Build history of the part. All positions in model axes, mm. Round coordinates to 2 decimals unless told otherwise and drop trailing zeros. Write each loop counter-clockwise with the first axis right and the second up, starting at its lowest first coordinate (ties: lowest second). Pieces come first, ordered by that corner, then holes. Notation, with made-up numbers: (-9, 36) -> (35, 36) arc R34 cw to (35, 73) -> close; hole circle Ø1 at (61.5, -39). An arc over 180 degrees is marked (long way). Answer in a Markdown table with one row per item.
```python
from build123d import *

# Parameters (mm, degrees)
F0_W        = 25.4
F0_H        = 25.4
F1_DEPTH    = 7.62
F2_R        = 5.08
F3_T1_DEPTH = 47.3970452561
F3_T3_DEPTH = 47.3970452561


# Not quite as in the source:
# - a fillet or chamfer that OpenCascade refuses, or shapes differently, is made with other operations: its cross-section is extruded or revolved along the edge and cut away or added


with BuildPart() as f1:
    # F0 (on Front) → F1 (new body)
    with BuildSketch(Plane.XZ):
        Rectangle(F0_W, F0_H)
    extrude(amount=F1_DEPTH)

    # F2
    f2_edges = [f1.edges().sort_by_distance(p)[0] for p in [
        (0, -7.62, 12.7),
        (-12.7, -7.62, 0),
        (12.7, -7.62, 0),
        (0, -7.62, -12.7),
    ]]
    fillet(f2_edges, radius=F2_R)

    # F3: fillet of radius 5.08 on 4 edges, made by hand

    # F3_s2 → F3_t1 (cut)
    with BuildSketch(Plane.YZ.offset(-23.6985226281)):
        with BuildLine():
            ThreePointArc((-2.54, -12.7), (-0.6805909488, -10.8405909488), (0, -8.3005909488))
            Line((0, -8.3005909488), (0, -12.7))
            Line((0, -12.7), (-2.54, -12.7))
        make_face()
        with BuildLine():
            ThreePointArc((0, 8.3005909488), (-0.6805909488, 10.8405909488), (-2.54, 12.7))
            Line((-2.54, 12.7), (0, 12.7))
            Line((0, 12.7), (0, 8.3005909488))
        make_face()
    extrude(amount=F3_T1_DEPTH, mode=Mode.SUBTRACT)

    # F3_s4 → F3_t3 (cut)
    with BuildSketch(Plane.XY.offset(-23.6985226281)):
        with BuildLine():
            ThreePointArc((-8.3005909488, 0), (-10.8405909488, -0.6805909488), (-12.7, -2.54))
            Line((-12.7, -2.54), (-12.7, 0))
            Line((-12.7, 0), (-8.3005909488, 0))
        make_face()
        with BuildLine():
            ThreePointArc((12.7, -2.54), (10.8405909488, -0.6805909488), (8.3005909488, 0))
            Line((8.3005909488, 0), (12.7, 0))
            Line((12.7, 0), (12.7, -2.54))
        make_face()
    extrude(amount=F3_T3_DEPTH, mode=Mode.SUBTRACT)


solid = f1.part
```
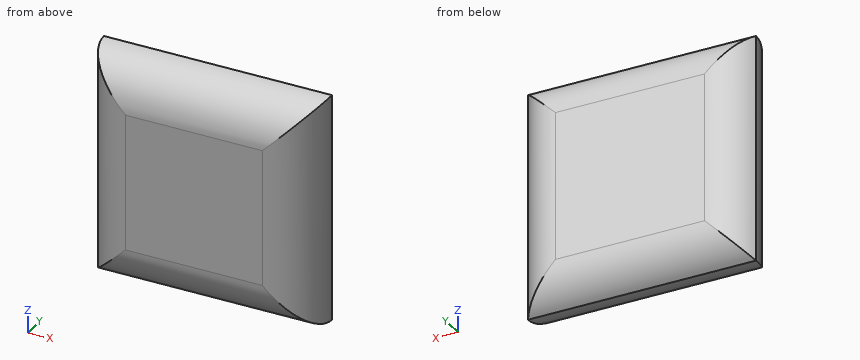
Q1. Saw through at C-C on y = -5.5. Write the cut outline in (x, z), plus the area to 3 significant figures.
A:
| item | result |
|---|---|
| outline | (-11.75, -11.75) -> (11.75, -11.75) -> (11.75, 11.75) -> (-11.75, 11.75) -> close |
| area | 552 mm² |
Q2. Saw through at D-D on y = -2. Write the cut outline in (x, z).
A:
| item | result |
|---|---|
| outline | (-12.34, -12.34) -> (12.34, -12.34) -> (12.34, 12.34) -> (-12.34, 12.34) -> close |
Q3. Wall check: line 1 (X direction, y = -6, z = -6.75); line 2 (X direction, y = -3.25, z = 0.75); line 3 (Y direction, x = 9, z = -9.5). Give the ranges that are in metal, low to high. Write a range as [from, to].
A:
| item | result |
|---|---|
| line 1 | [-11.34, 11.34] |
| line 2 | [-12.65, 12.65] |
| line 3 | [-7.26, -0.14] |
Q4. Saw through at A-A on x = -5.75. Write the cut outline in (y, z), plus the area to 3 significant figures.
A:
| item | result |
|---|---|
| outline | (-7.62, -7.62) arc R5.08 ccw to (-2.54, -12.7) arc R5.08 ccw to (0, -8.3) -> (0, 8.3) arc R5.08 ccw to (-2.54, 12.7) arc R5.08 ccw to (-7.62, 7.62) -> close |
| area | 176 mm² |
Q5. Drop flat-ended pins along their axis: P1, Ø1, axis at y = -5.5, z = 5, coming from the -X side; P2, Ø1, axis at y = -6.5, z = -2, coming from the +X side; P3, Ø3, axis at y = -1.5, z = -7.5, coming from the +X side. Give the stop position or say it passes through.
A:
| item | result |
|---|---|
| P1 | x = -12.06 |
| P2 | x = 11.34 |
| P3 | x = 12.7 |
Q6. Saw through at B-B on z = -1.75. Write the cut outline in (x, y).
A:
| item | result |
|---|---|
| outline | (-12.7, -2.54) arc R5.08 ccw to (-7.62, -7.62) -> (7.62, -7.62) arc R5.08 ccw to (12.7, -2.54) arc R5.08 ccw to (8.3, 0) -> (-8.3, 0) arc R5.08 ccw to start |
